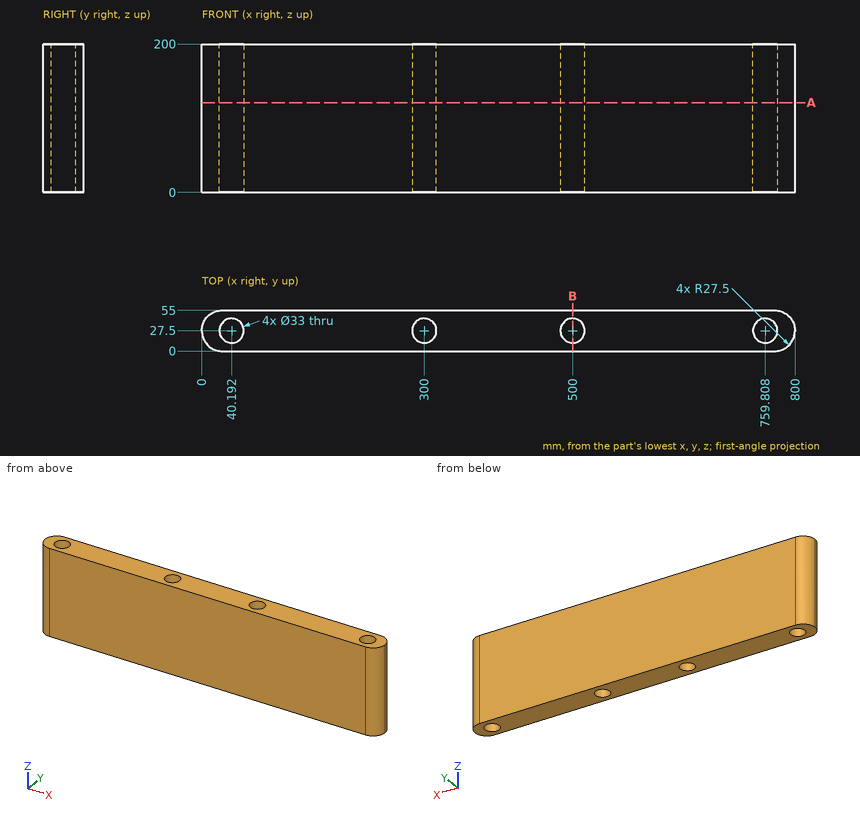
Source: three-view drawing plus pictorial views. Frame: mm from the lowest corner of the part. Coordinates: 2 decimals unless noted, no trailing zeros. Write each loop counter-clockwise with the first axis right and the second up, starting at its lowest first coordinate (ties: lowest second). Pieces come first, ordered by that corner, then holes. Notation, with made-up numbers: (-29, 38) - (4, 38) arc R30 cw to (4, 73) - close; hole circle Ø8 at (4, 41.5). An arc over 180 degrees is marked (long way). Return JSON: item names as keys, results as strings.
Item 1: Line query: L1, parallel to X at y = 27, z = 112 (1 decimal); L2, parallel to X at y = 35.5, z = 63; L3, parallel to Y at x = 300, z = 117. Output: solid intervals per line, ascending.
Completed:
{"L1": "x = 0 to 23.7, 56.7 to 283.5, 316.5 to 483.5, 516.5 to 743.3, 776.3 to 800", "L2": "x = 1.19 to 25.76, 54.62 to 285.57, 314.43 to 485.57, 514.43 to 745.38, 774.24 to 798.81", "L3": "y = 0 to 11, 44 to 55"}
Item 2: Section query A-A (z = 121). Count the separate pieces of the cut face and the enclosed holes in it, and give its area (3 significant figures).
Completed:
{"separate pieces": "1", "enclosed holes": "4", "area": "39,900 mm2"}
Item 3: Section query B-B (x = 500). Output: boundary loops of the cut face in (y, z).
Completed:
{"outline": "(0, 0) - (11, 0) - (11, 200) - (0, 200) - close; (44, 0) - (55, 0) - (55, 200) - (44, 200) - close"}
Item 4: Pin query (flat end, axial travel): pin 1 Ø5 at (y, z) = (31, 135.5) entering from +X; pin 2 Ø6 at (y, z) = (7.5, 46) entering from -X (1 decimal); pin 3 Ø1 at (y, z) = (7.5, 166) entering from -X. Return the tip coordinate at first contact, or that it passes through.
Completed:
{"pin 1": "stops at x = 799.98", "pin 2": "stops at x = 5.9", "pin 3": "stops at x = 8.11"}
